Autodesk Inventor part; units mm, degrees
ref_plane "Work Plane3" through (-5.6827, 14.6176, 2.5) normal (0, 0, 1) x (1, 0, 0)
ref_plane "YZ Plane" through (0, 0, 0) normal (1, 0, 0) x (0, 1, 0)
ref_plane "XZ Plane" through (0, 0, 0) normal (0, 1, 0) x (-1, 0, 0)
sketch "Sketch1" plane through (-3.508, -14.003, 0) normal (0, 0, 1) x (1, 0, 0)
  line L0 (-3.495, 25.7995) -> (-3.495, 3.5141)
  line L1 (28.511, 26.087) -> (28.511, 3.1543)
  line L2 (0.0191, 0) -> (25.3567, 0)
  line L3 (25.4878, 29.006) -> (-0.274, 29.006)
  arc A0 (-3.495, 3.5141) -> (0.0191, 0) centre (0.0191, 3.5141) ccw
  arc A1 (25.3567, 0) -> (28.511, 3.1543) centre (25.3567, 3.1543) ccw
  arc A2 (28.511, 25.9828) -> (25.4878, 29.006) centre (25.4878, 25.9827) ccw
  arc A3 (-0.274, 29.006) -> (-3.495, 25.7995) centre (-0.2885, 25.7995) ccw
  line L4 (9.8544, 29.006) -> (9.8544, 34.006) construction
  point P0 (12.6069, 14.6206)
  dimension "d0" = 5
sketch "Sketch3" plane through (0, 0, 0) normal (0, 0, 1) x (1, 0, 0)
  arc A0 (-5.6755, 17.1176) -> (-9.37, 13.4398) centre (-5.6922, 13.4398) ccw
  line L0 (-9.37, 13.4398) -> (-9.37, -12.1215)
  arc A1 (-9.37, -12.1215) -> (-5.3393, -16.1522) centre (-5.3393, -12.1215) ccw
  line L1 (-5.3393, -16.1522) -> (23.723, -16.1522)
  arc A2 (23.723, -16.1522) -> (27.3409, -12.5343) centre (23.723, -12.5343) ccw
  line L2 (27.3409, 13.7696) -> (27.3409, -12.5343)
  arc A3 (27.3409, 13.65) -> (23.8733, 17.1176) centre (23.8733, 13.65) ccw
  line L3 (23.8733, 17.1176) -> (-5.6755, 17.1176)
  point P0 (0, 0)
  point P1 (25.003, 11.9798)
  point P2 (9.0989, 0.6176)
extrude "Extrusion1" add sketch "Sketch3" along normal blind 7.886
shell "Shell1" thickness 2.5 removed faces 1 at (4.2862, 6.0277, 7.886)
ref_plane "Work Plane3" through (-5.6827, 14.6176, 2.5) normal (0, 0, 1) x (1, 0, 0)
sketch "Sketch4" plane through (-5.6827, 14.6176, 2.5) normal (0, 0, 1) x (1, 0, 0)
  point P0 (5.6827, -14.6176)
extrude "Extrusion2" cut sketch "Sketch1" along normal blind 21
sketch "Sketch5" plane through (-5.6827, 14.6176, 2.5) normal (0, 0, 1) x (1, 0, 0)
  arc A0 (0.3621, 0) -> (-1.1873, -1.9071) centre (1.8862, -2.8211) ccw
  line L0 (0.3621, 0) -> (0, 0)
  arc A1 (0, 0) -> (-1.1873, -1.1778) centre (-0.0094, -1.1778) ccw
  line L1 (-1.1873, -1.1778) -> (-1.1873, -1.9071)
  arc A2 (-1.1873, -26.0642) -> (0.6634, -28.2698) centre (2.1939, -25.1065) ccw
  line L2 (-1.1873, -26.0642) -> (-1.1873, -26.7391)
  arc A3 (-1.1873, -26.7391) -> (0.3435, -28.2698) centre (0.3435, -26.7391) ccw
  line L3 (0.3435, -28.2698) -> (0.6634, -28.2698)
  arc A4 (28.9771, -28.2698) -> (30.5236, -26.4645) centre (27.5315, -25.4663) ccw
  line L4 (28.9771, -28.2698) -> (29.4057, -28.2698)
  arc A5 (29.4057, -28.2698) -> (30.5236, -27.1519) centre (29.4057, -27.1519) ccw
  line L5 (30.5236, -27.1519) -> (30.5236, -26.4645)
  arc A6 (30.5236, -1.6612) -> (29.1395, 0) centre (27.6625, -2.6379) ccw
  line L6 (30.5236, -1.6612) -> (30.5236, -0.9676)
  arc A7 (30.5236, -0.9676) -> (29.556, 0) centre (29.556, -0.9676) ccw
  line L7 (29.556, 0) -> (29.1395, 0)
  point P0 (5.6827, -14.6176)
extrude "Extrusion3" add sketch "Sketch5" along normal up to surface (5.386 mm away)
sketch "Sketch6" plane through (-5.6827, 14.6176, 2.5) normal (0, 0, 1) x (1, 0, 0)
  arc A0 (27.5315, -28.6206) -> (30.6857, -25.4663) centre (27.5315, -25.4663) ccw
  line L0 (2.1939, -28.6206) -> (27.5315, -28.6206)
  arc A1 (-1.3203, -25.1065) -> (2.1939, -28.6206) centre (2.1939, -25.1065) ccw
  line L1 (-1.3203, -2.8211) -> (-1.3203, -25.1065)
  arc A2 (1.9007, 0.3854) -> (-1.3203, -2.8211) centre (1.8862, -2.8211) ccw
  line L2 (27.6625, 0.3854) -> (1.9007, 0.3854)
  arc A3 (30.6857, -2.6378) -> (27.6625, 0.3854) centre (27.6625, -2.6379) ccw
  line L3 (30.6857, -25.4663) -> (30.6857, -2.6378)
  point P0 (5.6827, -14.6176)
extrude "Extrusion4" add sketch "Sketch6" against normal up to surface (2.5 mm away)
sketch "Sketch7" plane through (-5.6827, 14.6176, 2.5) normal (0, 0, 1) x (1, 0, 0)
  arc A0 (27.5315, -28.6206) -> (30.6857, -25.4663) centre (27.5315, -25.4663) ccw
  line L0 (30.6857, -2.6378) -> (30.6857, -25.4663)
  arc A1 (30.6857, -2.6378) -> (27.6625, 0.3854) centre (27.6625, -2.6379) ccw
  line L1 (1.9007, 0.3854) -> (27.6625, 0.3854)
  arc A2 (1.9007, 0.3854) -> (-1.3203, -2.8211) centre (1.8862, -2.8211) ccw
  line L2 (-1.3203, -25.1065) -> (-1.3203, -2.8211)
  arc A3 (-1.3203, -25.1065) -> (2.1939, -28.6206) centre (2.1939, -25.1065) ccw
  line L3 (27.5315, -28.6206) -> (2.1939, -28.6206)
  arc A4 (1.8968, -1.1146) -> (0.1797, -2.8211) centre (1.8862, -2.8211) ccw
  line L4 (1.8968, -1.1146) -> (27.6625, -1.1146)
  arc A5 (29.1857, -2.6379) -> (27.6625, -1.1146) centre (27.6625, -2.6379) ccw
  line L5 (29.1857, -2.6379) -> (29.1857, -25.4663)
  arc A6 (27.5315, -27.1206) -> (29.1857, -25.4663) centre (27.5315, -25.4663) ccw
  line L6 (27.5315, -27.1206) -> (2.1939, -27.1206)
  arc A7 (0.1797, -25.1065) -> (2.1939, -27.1206) centre (2.1939, -25.1065) ccw
  line L7 (0.1797, -25.1065) -> (0.1797, -2.8211)
  point P0 (5.6827, -14.6176)
  dimension "d11" = 1.5
extrude "Extrusion5" [suppressed]
fillet "Fillet1" radius 2 8 edges at (26.3252, 16.102, 0) (27.3409, 0.5579, 0) (26.2812, -15.0926, 0) (9.1919, -16.1522, 0) (-8.1894, -14.9717, 0) (-9.37, 0.6592, 0) (-8.2869, 16.0463, 0) (9.0989, 17.1176, 0)
sketch "Sketch9" plane through (-5.6827, 14.6176, 2.5) normal (0, 0, 1) x (1, 0, 0)
  arc A0 (27.5315, -28.6206) -> (30.6857, -25.4663) centre (27.5315, -25.4663) ccw
  line L0 (30.6857, -2.6378) -> (30.6857, -25.4663)
  arc A1 (30.6857, -2.6378) -> (27.6625, 0.3854) centre (27.6625, -2.6379) ccw
  line L1 (1.9007, 0.3854) -> (27.6625, 0.3854)
  arc A2 (1.9007, 0.3854) -> (-1.3203, -2.8211) centre (1.8862, -2.8211) ccw
  line L2 (-1.3203, -25.1065) -> (-1.3203, -2.8211)
  arc A3 (-1.3203, -25.1065) -> (2.1939, -28.6206) centre (2.1939, -25.1065) ccw
  line L3 (27.5315, -28.6206) -> (2.1939, -28.6206)
  point P0 (5.6827, -14.6176)
extrude "Extrusion7" cut sketch "Sketch9" against normal blind 1.6
properties part number "GoPro_Cap_Lens"
Can you work these out from the model? Positions are in its coordinate system, mm. A direction names the side the tool comes from. Coordinates: 2 decimals unless noted, no trailing zeros. Write each loop counter-clockwise with the first axis right and the second up, starting at its lowest first coordinate (ties: lowest second). Pieces come first, ordered by that corner, then holes.
Q1. Which directions (+Z, -Z, +X, -X, +Y, -Y) give clear straight access to the entire face, cutting with the end or side of a thin tool? Please do faces 1 (the face through (26.298, 16.129, 4.902)), 2 (the face through (-6.3, 13.8, 5.2)).
Results found:
face 1: +Z, -Z, +X, +Y
face 2: +Z
Q2. Imagine slicing it at B-B, the plane y = 2.5. List the corners of the cut face in (x, z) for me, plus the area to 3 significant figures.
Results found:
outline: (-9.37, 2) arc R2 ccw to (-7.37, 0) - (25.34, 0) arc R2 ccw to (27.34, 2) - (27.34, 7.89) - (25, 7.89) - (25, 0.9) - (-7, 0.9) - (-7, 7.89) - (-9.37, 7.89) - close
area: 64.2 mm2
Q3. Please list where these lines run through material, in increasing order: L1, parallel to Y at x = 20.5, z = 4.25; L2, parallel to X at y = 4, z = 2; L3, parallel to Z at x = 25.5, y = -5.5.
Results found:
L1: y = -16.15 to -14, 15 to 17.12
L2: x = -9.37 to -7, 25 to 27.34
L3: z = 0.01 to 7.89
Q4. Imagine slicing it at C-C, the plane z = 3.25. List the corners of the cut face in (x, y) for me, plus the area to 3 significant figures.
Results found:
outline: (-9.37, -12.12) arc R4.03 ccw to (-5.34, -16.15) - (23.72, -16.15) arc R3.62 ccw to (27.34, -12.53) - (27.34, 13.65) arc R3.47 ccw to (23.87, 17.12) - (-5.68, 17.12) arc R3.68 ccw to (-9.37, 13.44) - close; hole (-7, -10.49) arc R3.51 ccw to (-6.87, -11.45) arc R3.51 ccw to (-5.02, -13.65) arc R3.51 ccw to (-3.49, -14) - (21.85, -14) arc R3.15 ccw to (23.29, -13.65) arc R3.15 ccw to (24.84, -11.85) arc R3.15 ccw to (25, -10.85) - (25, 12.08) arc R3.02 ccw to (24.84, 12.96) arc R3.02 ccw to (23.46, 14.62) arc R3.02 ccw to (21.98, 15) - (-3.78, 15) arc R3.21 ccw to (-5.32, 14.62) arc R3.21 ccw to (-6.87, 12.71) arc R3.21 ccw to (-7, 11.8) - close
area: 290 mm2
Q5. For P1, Ø12, axis at x = 1.5, y = -12, coming from the +Z side; P2, Ø0.8, axis at x = 5, z = 1.5, coming from the +Y side; P3, Ø14.5, axis at x = 11, y = -3, coming from the +Z side, each with a flat end and sliding along its axis, tell me the tip position at first contact or that it passes through.
Results found:
P1: stops at z = 7.89
P2: stops at y = 17.12
P3: stops at z = 0.9
Q6. If we mould it in two halves opening along Y, with no side actions, what happens to faces 3 (the face through (26.77, 0.74, 0.6)), 4 (the face through (24.255, -12.888, 5.155)), 5 (the face through (8.892, 16.547, 0.601))? For each: +Y half, -Y half, draft (parallel to the pull), parting line (faces both ways), or undercut.
Results found:
face 3: draft
face 4: undercut
face 5: +Y half
Q7. Imagine slicing it at A-A, the plane x = 15. List the corners of the cut face in (y, z) for me.
Results found:
outline: (-16.15, 2) arc R2 ccw to (-14.15, 0) - (15.12, 0) arc R2 ccw to (17.12, 2) - (17.12, 7.89) - (15, 7.89) - (15, 0.9) - (-14, 0.9) - (-14, 7.89) - (-16.15, 7.89) - close
